```python
from build123d import *

# Parameters (mm, degrees)
SKETCH_1_W        = 120
SKETCH_1_H        = 70
SKETCH_1_W_2      = 74
SKETCH_1_H_2      = 50
EXTRUDE_1_DEPTH   = 2.5
FILLET_1_R        = 5.5
EXTRUDE_1_2_DEPTH = 4


with BuildPart() as part:
    # 草图1 → Extrude 1 (new body)
    with BuildSketch(Plane.XY):
        with Locations((8.671272412, 0.068259877)):
            Rectangle(SKETCH_1_W, SKETCH_1_H)
        with Locations((7.671272412, 0.068259877)):
            Rectangle(SKETCH_1_W_2, SKETCH_1_H_2, mode=Mode.SUBTRACT)
    extrude(amount=EXTRUDE_1_DEPTH)

    # 圆角1
    fillet_1_edges = [part.edges().sort_by_distance(p)[0] for p in [
        (-51.328727588, 35.068259877, 1.25),
        (68.671272412, 35.068259877, 1.25),
        (68.671272412, -34.931740123, 1.25),
        (-51.328727588, -34.931740123, 1.25),
    ]]
    fillet(fillet_1_edges, radius=FILLET_1_R)

    # 草图2 → Extrude 1 2 (add)
    with BuildSketch(Plane(origin=(0, 0, 0), x_dir=(-1, 0, 0), z_dir=(0, 0, -1))):
        with BuildLine():
            Line((-63.021272412, 32.418259877), (45.678727588, 32.418259877))
            ThreePointArc((45.678727588, 32.418259877), (48.082890644, 31.422422933), (49.078727588, 29.018259877))
            Line((49.078727588, 29.018259877), (49.078727588, -28.881740123))
            ThreePointArc((49.078727588, -28.881740123), (48.082890644, -31.285903179), (45.678727588, -32.281740123))
            Line((45.678727588, -32.281740123), (-63.021272412, -32.281740123))
            ThreePointArc((-63.021272412, -32.281740123), (-65.425435468, -31.285903179), (-66.421272412, -28.881740123))
            Line((-66.421272412, -28.881740123), (-66.421272412, 29.018259877))
            ThreePointArc((-66.421272412, 29.018259877), (-65.425435468, 31.422422933), (-63.021272412, 32.418259877))
        make_face()
        with BuildLine():
            Line((-63.021272412, 30.418259877), (45.678727588, 30.418259877))
            ThreePointArc((45.678727588, 30.418259877), (46.668677082, 30.008209371), (47.078727588, 29.018259877))
            Line((47.078727588, 29.018259877), (47.078727588, -28.881740123))
            ThreePointArc((47.078727588, -28.881740123), (46.668677082, -29.871689616), (45.678727588, -30.281740123))
            Line((45.678727588, -30.281740123), (-63.021272412, -30.281740123))
            ThreePointArc((-63.021272412, -30.281740123), (-64.011221906, -29.871689616), (-64.421272412, -28.881740123))
            Line((-64.421272412, -28.881740123), (-64.421272412, 29.018259877))
            ThreePointArc((-64.421272412, 29.018259877), (-64.011221906, 30.008209371), (-63.021272412, 30.418259877))
        make_face(mode=Mode.SUBTRACT)
    extrude(amount=EXTRUDE_1_2_DEPTH)


solid = part.part
```
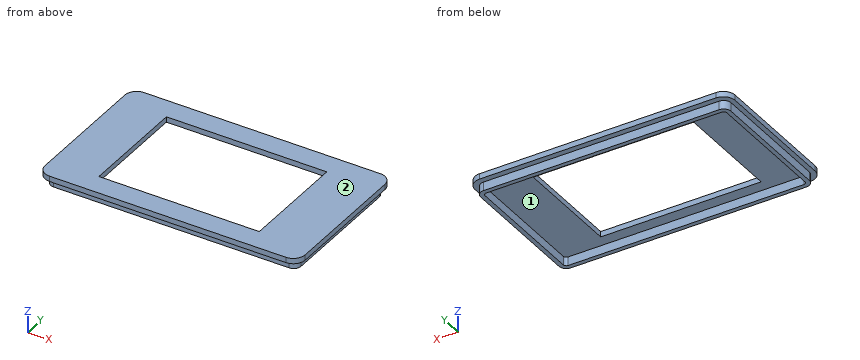
Model file for the job. Use its own axes, mm. Face numbers are marked on the shaded views. Give positions to 0.01 mm unless a question says otherwise; leave off trailing zeros. Order: outer loops, then holes, each group sorted by start corner. A loop starts at its lowest first (then second) coordinate and runs counter-clockwise, first axis right, second up.
1) Wall check: probe 1 along X at (y, z) = (14, -1.75); probe 2 along Y at (x, z) = (14, 0.5); probe 3 along Y at (x, z) = (57.5, -3.5). Give the ranges that are in metal, low to high.
2) Saw through at B-B, the plane x = 14.5. Write the cut outline in (y, z).
3) Pin check, flat tips, straight feed: pin 1 (2 mm diameter, centred on x = -8.5, z = -2, fed in from +Y); pin 2 (2 mm diameter, centred on x = 1, z = -1.5, fed in from -Y); pin 3 (5 mm diameter, centred on x = -27, y = -21.5, fed in from -Z). Stop position of each tip, or through.
4) Mould opens along X. For the marked faces 1 and 2 say: +X half, -X half, draft (parallel to the pull), parting line (faces both ways), or undercut.
5) Saw through at C-C, the plane z = 1. Write the cut outline in (x, y), then the cut area to 3 significant figures.
6) Saw through at A-A, the plane y = 0. Write the cut outline in (x, z).
Computed:
1. probe 1: x = -49.08 to -47.08, 64.42 to 66.42
1. probe 2: y = -34.93 to -24.93, 25.07 to 35.07
1. probe 3: y = -32.28 to -30.28, 30.42 to 32.42
2. outline: (-34.93, 0) - (-32.28, 0) - (-32.28, -4) - (-30.28, -4) - (-30.28, 0) - (-24.93, 0) - (-24.93, 2.5) - (-34.93, 2.5) - close; (25.07, 0) - (30.42, 0) - (30.42, -4) - (32.42, -4) - (32.42, 0) - (35.07, 0) - (35.07, 2.5) - (25.07, 2.5) - close
3. pin 1: stops at y = 32.42
3. pin 2: stops at y = -32.28
3. pin 3: stops at z = 0
4. face 1: undercut
4. face 2: draft
5. outline: (-51.33, -29.43) arc R5.5 ccw to (-45.83, -34.93) - (63.17, -34.93) arc R5.5 ccw to (68.67, -29.43) - (68.67, 29.57) arc R5.5 ccw to (63.17, 35.07) - (-45.83, 35.07) arc R5.5 ccw to (-51.33, 29.57) - close; hole (-29.33, -24.93) - (44.67, -24.93) - (44.67, 25.07) - (-29.33, 25.07) - close
5. area: 4,670 mm2
6. outline: (-51.33, 0) - (-49.08, 0) - (-49.08, -4) - (-47.08, -4) - (-47.08, 0) - (-29.33, 0) - (-29.33, 2.5) - (-51.33, 2.5) - close; (44.67, 0) - (64.42, 0) - (64.42, -4) - (66.42, -4) - (66.42, 0) - (68.67, 0) - (68.67, 2.5) - (44.67, 2.5) - close
